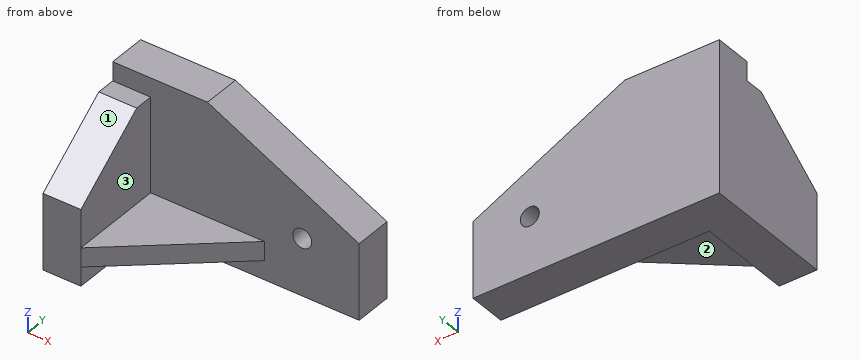
```python
from build123d import *

# Parameters (mm, degrees)
F0_W      = 65
F0_H      = 40
F1_DEPTH  = 35
F2_W      = 55
F2_H      = 40
F3_DEPTH  = 25
F4_W      = 5
F4_H      = 5
F5_DEPTH  = 65.001
F6_R      = 2.5
F7_DEPTH  = 10.001
F9_DEPTH  = 65.001
F11_DEPTH = 35.001
F12_W     = 30
F12_H     = 5
F13_DEPTH = 25
F15_DEPTH = 10.001


with BuildPart() as f1:
    # F0 (on Front) → F1 (new body)
    with BuildSketch(Plane.XZ):
        Rectangle(F0_W, F0_H)
    extrude(amount=F1_DEPTH)

    # F2 (on face) → F3 (cut)
    with BuildSketch(Plane.XZ.offset(35)):
        with Locations((5, 0)):
            Rectangle(F2_W, F2_H)
    extrude(amount=-F3_DEPTH, mode=Mode.SUBTRACT)

    # F4 (on face) → F5 (cut, through all)
    with BuildSketch(Plane(origin=(-32.5, 0, 0), x_dir=(0, -1, 0), z_dir=(-1, 0, 0))):
        with Locations((12.5, 17.5)):
            Rectangle(F4_W, F4_H)
    extrude(amount=-F5_DEPTH, mode=Mode.SUBTRACT)

    # F6 (on face) → F7 (cut, through all)
    with BuildSketch(Plane.XZ.offset(10)):
        with Locations((17.5, -5)):
            Circle(F6_R)
    extrude(amount=-F7_DEPTH, mode=Mode.SUBTRACT)

    # F8 (on face) → F9 (cut, through all)
    with BuildSketch(Plane(origin=(-32.5, 0, 0), x_dir=(0, -1, 0), z_dir=(-1, 0, 0))):
        Polygon((15, 20), (15, 15), (35, 0), (35, 20), align=None)
    extrude(amount=-F9_DEPTH, mode=Mode.SUBTRACT)

    # F10 (on face) → F11 (cut, through all)
    with BuildSketch(Plane(origin=(0, 0, 0), x_dir=(-1, 0, 0), z_dir=(0, 1, 0))):
        Polygon((7.5, 20), (-32.5, 20), (-32.5, 0), align=None)
    extrude(amount=-F11_DEPTH, mode=Mode.SUBTRACT)

    # F12 (on face) → F13 (join)
    with BuildSketch(Plane.XZ.offset(10)):
        with Locations((-7.5, -12.5)):
            Rectangle(F12_W, F12_H)
    extrude(amount=F13_DEPTH)

    # F14 (on face) → F15 (cut, through all)
    with BuildSketch(Plane.XY.offset(-10)):
        Polygon((7.5, -10), (-22.5, -35), (7.5, -35), align=None)
    extrude(amount=-F15_DEPTH, mode=Mode.SUBTRACT)


solid = f1.part
```
Geometry: final body of the model. Coordinates: model frame, mm. Face numbers are marked on the shaded views. A direction names the side the tool comes from. Round coordinates to 2 decimals unless told otherwise and drop trailing zeros. Order: outer loops, then holes, each group sorted by start corner. A loop starts at its lowest first (then second) coordinate and runs counter-clockwise, first axis right, second up. Notation, with made-up numbers: (-25.75, 47.25) - (-20.75, 47.25) arc R29 cw to (-20.75, 85.25) - close; hole circle Ø4 at (-37, 25.25). An arc over 180 degrees is marked (long way). Write item = value, one per line. Start each with the question number.
Q1. Ray query, line 1 (Y direction, x = -11.5, z = 10); line 2 (X direction, y = -33.5, z = -4); line 3 (Z direction, x = -9, y = -17.5). Return the intervals inside material, ascending. Write a range as from..to.
Q2. Pin query (flat end, axial travel): pin 1 (6 mm diameter, centred on y = -23, z = -3.5, fed in from +X); pin 2 (20 mm diameter, centred on x = -5, y = -22.5, fed in from -Z); pin 3 (12.5 mm diameter, centred on x = -12, y = -17.5, fed in from +Z). Return the tip coordinate at first contact, or that it passes through.
Q3. Cut plane A-A on x = -13.5. Return the cut outline in (y, z), and give its area (4 significant figures).
Q4. Access query for the marked faces 1, 2 and 3. Directions: +Z, -Z, +X, -X, +Y, -Y. A direction counts if a zero-diameter tool reaches every point of the face in a straight line with its end or side. Return the directions, or none.
Q5. Cut plane B-B on y = -32. Return the cut outline in (x, z), and give its area (4 significant figures).
Q6. Cut plane C-C on z = -5. Return the cut outline in (x, y).
Q7. Cut plane D-D on x = 17.5. Return the cut outline in (y, z).
Outcome:
q1.line_1 = -10..0
q1.line_2 = -32.5..-22.5
q1.line_3 = -15..-10
q2.pin_1 = -22.5
q2.pin_2 = -15
q2.pin_3 = -10
q3.outline = (-27.5, -15) - (-10, -15) - (-10, -20) - (0, -20) - (0, 20) - (-10, 20) - (-10, -10) - (-27.5, -10) - close
q3.area = 487.5 mm^2
q4.face_1 = +Z, +X, -X, -Y
q4.face_2 = -Z, +X, -Y
q4.face_3 = +Z, +X, -Y
q5.outline = (-32.5, -20) - (-22.5, -20) - (-22.5, -15) - (-18.9, -15) - (-18.9, -10) - (-22.5, -10) - (-22.5, 2.25) - (-32.5, 2.25) - close
q5.area = 240.5 mm^2
q6.outline = (-32.5, -35) - (-22.5, -35) - (-22.5, -10) - (15, -10) - (15, 0) - (-32.5, 0) - close; (20, -10) - (32.5, -10) - (32.5, 0) - (20, 0) - close
q7.outline = (-10, -20) - (0, -20) - (0, -7.5) - (-10, -7.5) - close; (-10, -2.5) - (0, -2.5) - (0, 7.5) - (-10, 7.5) - close
